```python
from build123d import *

# Parameters (mm, degrees)
F2_R     = 1.905
F3_DEPTH = 4.4958
F4_R     = 0.0508


with BuildPart() as f1:
    # F0 (on Right) → F1 (revolve)
    with BuildSketch(Plane.YZ):
        Polygon((2.8448, 0), (1.905, 0), (1.905, -5.588), (2.3241, -5.588), (2.3241, -11.2014), (2.8448, -11.2014), (2.8448, -10.2616), (3.0988, -10.2616), (3.0988, -10.0076), (2.8448, -10.0076), align=None)
    revolve(axis=Axis((0, 0, -5.6007), (0, 0, -1)))

    # F2 (on face) → F3 (cut)
    with BuildSketch(Plane.XY):
        with BuildLine():
            ThreePointArc((2.7893779952, 0.5588), (0, 2.8448), (-2.7893779952, 0.5588))
            Line((-2.7893779952, 0.5588), (-2.0828, 0.5588))
            Line((-2.0828, 0.5588), (-2.0828, -0.254))
            Line((-2.0828, -0.254), (-2.8334380247, -0.254))
            ThreePointArc((-2.8334380247, -0.254), (0, -2.8448), (2.8334380247, -0.254))
            Line((2.8334380247, -0.254), (2.0828, -0.254))
            Line((2.0828, -0.254), (2.0828, 0.5588))
            Line((2.0828, 0.5588), (2.7893779952, 0.5588))
        make_face()
        Circle(F2_R, mode=Mode.SUBTRACT)
    extrude(amount=-F3_DEPTH, mode=Mode.SUBTRACT)

    # F4
    f4_edges = [f1.edges().sort_by_distance(p)[0] for p in [
        (-2.789378, 0.5588, -2.2479),
        (-2.0828, 0.5588, -2.2479),
        (-2.0828, -0.254, -2.2479),
        (-2.833438, -0.254, -2.2479),
        (2.0828, -0.254, -2.2479),
        (2.833438, -0.254, -2.2479),
        (2.789378, 0.5588, -2.2479),
        (2.0828, 0.5588, -2.2479),
    ]]
    fillet(f4_edges, radius=F4_R)


solid = f1.part
```
Check sheet for the modelled part. Datum: model origin and axes. Units: mm. A direction names the side the tool comes from. Round coordinates to 2 decimals unless told otherwise and drop trailing zeros. Loops run counter-clockwise (first coordinate to the right, second up) from the corner with the lowest first, then second, coordinate; pieces in that order, holes last. Notation, with made-up numbers: (83.25, 57.25) - (101.25, 57.25) arc R15 cw to (101.25, 77.25) - close; hole circle Ø9 at (70, -23). An arc over 180 degrees is marked (long way). Write item = value, one per line. Start each with the question number.
Q1. Section check A-A (y = 0). Record the boundary of the cut face in (x, z) (3 decimals).
Q2. Thickness scan on L1, parallel to X at y = 0, z = -4.95 (3 decimals); L2, parallel to X at y = 0, z = -1.25; L3, parallel to Z at x = -1, y = -1.75. Record the ranges inside material, lowest first.
Q3. Section check C-C (x = 1.5). Record the boundary of the cut face in (y, z), plus the area to 3 significant figures.
Q4. Access from +Z, -Z, +X, -X, +Y, -Y to the whole of each face (thin tool, end or side, straight path). Record for faces 4 (the face through (0.572, 1.817, -5.05)), 5 (the face through (-2.777, -0.617, -10.725)).
Q5. Section check D-D (z = -8). Record the boundary of the cut face in (x, y).
Q6. Section check B-B (z = -3.5). Record the boundary of the cut face in (x, y), plus the area to 3 significant figures.
Q7. Release check for a two-part mould opening along Y. For faces 1 (the face through (0.9, 2.7, -7.2)), 2 (the face through (2, -1, -4.496)), 3 (the face through (-2.27, -0.5, -8.43)) record: pulls with the +Y half, pulls with the -Y half, needs draft (parallel to the pull), parting line crosses it, or undercut.
Q8. Depth check by flat-ended pin: P1, Ø3, axis at x = 1, y = 2, coming from the +Z side; P2, Ø0.7, axis at x = -2.5, z = -3, coming from the +Y side; P3, Ø2, axis at y = 2.5, z = -6.5, coming from the +X side. Enter the tip coordinate at first touch or a pass-through.
Derived:
q1.outline = (-3.099, -10.262) - (-2.845, -10.262) - (-2.845, -11.201) - (-2.324, -11.201) - (-2.324, -5.588) - (-1.905, -5.588) - (-1.905, -4.496) - (-2.083, -4.496) - (-2.083, 0) - (-2.845, 0) - (-2.845, -10.008) - (-3.099, -10.008) - close; (1.905, -5.588) - (2.324, -5.588) - (2.324, -11.201) - (2.845, -11.201) - (2.845, -10.262) - (3.099, -10.262) - (3.099, -10.008) - (2.845, -10.008) - (2.845, 0) - (2.083, 0) - (2.083, -4.496) - (1.905, -4.496) - close
q2.L1 = -2.845 to -1.905, 1.905 to 2.845
q2.L2 = -2.84 to -2.08, 2.08 to 2.84
q2.L3 = -5.59 to -4.5
q3.outline = (-2.71, -10.26) - (-2.42, -10.26) - (-2.42, -11.2) - (-1.78, -11.2) - (-1.78, -5.59) - (-1.17, -5.59) - (-1.17, -4.5) - (-2.42, -4.5) - (-2.42, -10.01) - (-2.71, -10.01) - close; (1.17, -5.59) - (1.78, -5.59) - (1.78, -11.2) - (2.42, -11.2) - (2.42, -10.26) - (2.71, -10.26) - (2.71, -10.01) - (2.42, -10.01) - (2.42, -4.5) - (1.17, -4.5) - close
q3.area = 10.1 mm^2
q4.face_4 = +Z, -Z
q4.face_5 = -Z
q5.outline = circle Ø5.69 at (0, 0); hole circle Ø4.65 at (0, 0)
q6.outline = (-2.84, -0.21) arc R0.05 ccw to (-2.79, -0.25) - (-2.13, -0.25) arc R0.05 ccw to (-2.08, -0.2) - (-2.08, 0.51) arc R0.05 ccw to (-2.13, 0.56) - (-2.75, 0.56) arc R0.05 ccw to (-2.8, 0.52) arc R2.84 ccw to start; (2.08, -0.2) arc R0.05 ccw to (2.13, -0.25) - (2.79, -0.25) arc R0.05 ccw to (2.84, -0.21) arc R2.84 ccw to (2.8, 0.52) arc R0.05 ccw to (2.75, 0.56) - (2.13, 0.56) arc R0.05 ccw to (2.08, 0.51) - close
q6.area = 1.21 mm^2
q7.face_1 = parting line crosses it
q7.face_2 = needs draft
q7.face_3 = undercut
q8.P1 = -4.5
q8.P2 = 0.56
q8.P3 = 2.42
